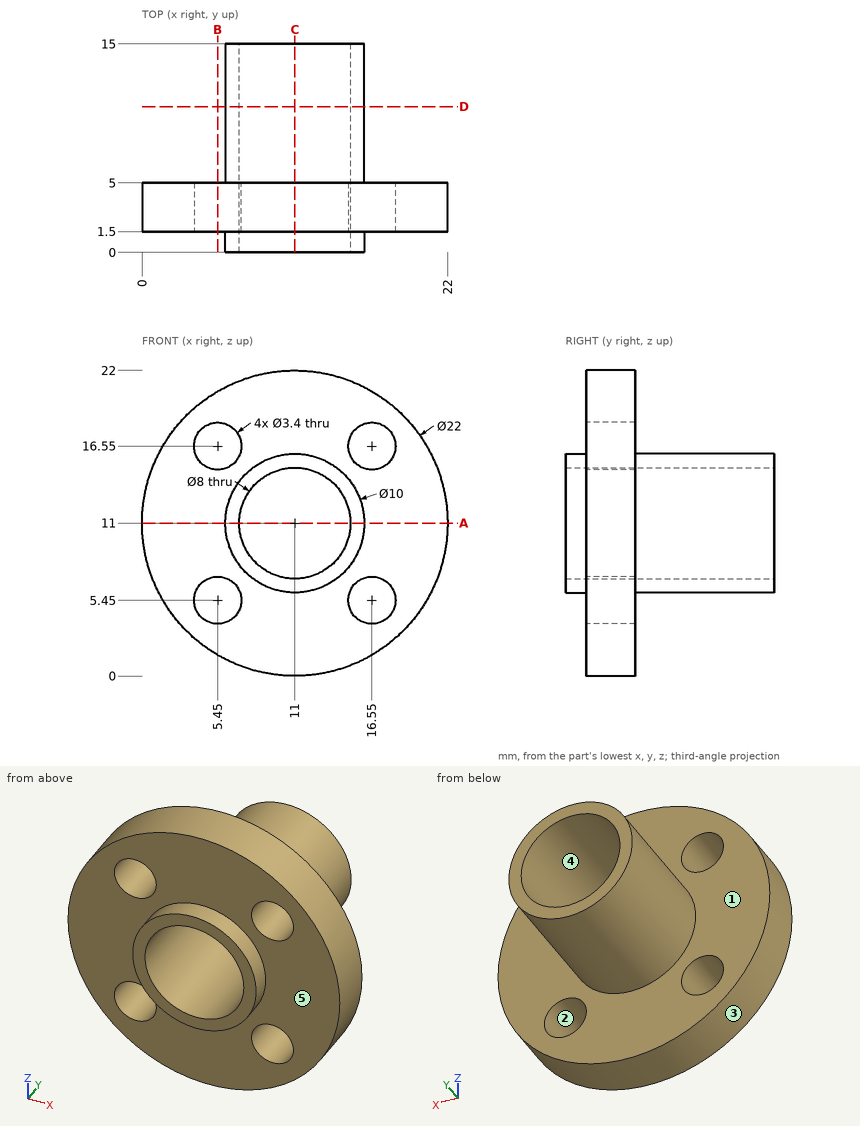
Source: three-view drawing plus pictorial views. Frame: mm from the lowest corner of the part. A direction names the side the tool comes from. Round coordinates to 2 decimals unless told otherwise and drop trailing zeros. Order: outer loops, then holes, each group sorted by start corner. A loop starts at its lowest first (then second) coordinate and runs counter-clockwise, first axis right, second up. Notation, with made-up numbers: (-31.5, -30.5) -> (17.5, -30.5) arc R8 cw to (17.5, -24.5) -> close; hole circle Ø5 at (-18, 53). An arc over 180 degrees is marked (long way). Use one line per item in the form item = value.
(1) Ray query, probe 1 along X at (y, z) = (3.35, 16.55); probe 2 along Z at (x, y) = (11, 2.25); probe 3 along X at (y, z) = (5.75, 11). Return the intervals inside material, ascending. Write a range as [from, to].
Results list:
probe_1 = [1.5, 3.75], [7.15, 14.85], [18.25, 20.5]
probe_2 = [0, 7], [15, 22]
probe_3 = [6, 7], [15, 16]
(2) Section D-D on y = 10.5. Return loops of the section in (x, z).
Results list:
outline = circle Ø10 at (11, 11); hole circle Ø8 at (11, 11)
(3) Section B-B on x = 5.45. Return loops of the section in (y, z), and give its area (3 significant figures).
Results list:
outline = (1.5, 1.5) -> (5, 1.5) -> (5, 3.75) -> (1.5, 3.75) -> close; (1.5, 7.15) -> (5, 7.15) -> (5, 14.85) -> (1.5, 14.85) -> close; (1.5, 18.25) -> (5, 18.25) -> (5, 20.5) -> (1.5, 20.5) -> close
area = 42.7 mm^2
(4) Section A-A on z = 11. Return loops of the section in (x, y).
Results list:
outline = (0, 1.5) -> (6, 1.5) -> (6, 0) -> (7, 0) -> (7, 15) -> (6, 15) -> (6, 5) -> (0, 5) -> close; (15, 0) -> (16, 0) -> (16, 1.5) -> (22, 1.5) -> (22, 5) -> (16, 5) -> (16, 15) -> (15, 15) -> close
(5) Draft query along Z for the marked faces 3, 4 and 5. Return one class per face: pulls with the +Z half, pulls with the -Z half, needs draft (parallel to the pull), parting line crosses it, or undercut.
Results list:
face_3 = parting line crosses it
face_4 = undercut
face_5 = needs draft
(6) Section C-C on x = 11. Return loops of the section in (y, z).
Results list:
outline = (0, 6) -> (1.5, 6) -> (1.5, 0) -> (5, 0) -> (5, 6) -> (15, 6) -> (15, 7) -> (0, 7) -> close; (0, 15) -> (15, 15) -> (15, 16) -> (5, 16) -> (5, 22) -> (1.5, 22) -> (1.5, 16) -> (0, 16) -> close
(7) Access query for the marked faces 1 and 2. Directions: +Z, -Z, +X, -X, +Y, -Y. A direction counts if a zero-diameter tool reaches every point of the face in a straight line with its end or side. Return the directions, or none.
Results list:
face_1 = +Y
face_2 = +Y, -Y
(8) First-contact query: pin 1 Ø2 at (x, z) = (16.55, 16.55) entering from +Y; pin 2 Ø1.5 at (x, y) = (14, 11.5) entering from +Z; pin 3 Ø5.5 at (x, z) = (5.45, 16.55) entering from +Y; pin 4 Ø4 at (x, y) = (5, 6.5) entering from -Z. Flat tips, straight axial feed; report the tip coordinate or a pass-through.
Results list:
pin_1 = through
pin_2 = 15.47
pin_3 = 5
pin_4 = 1.04
